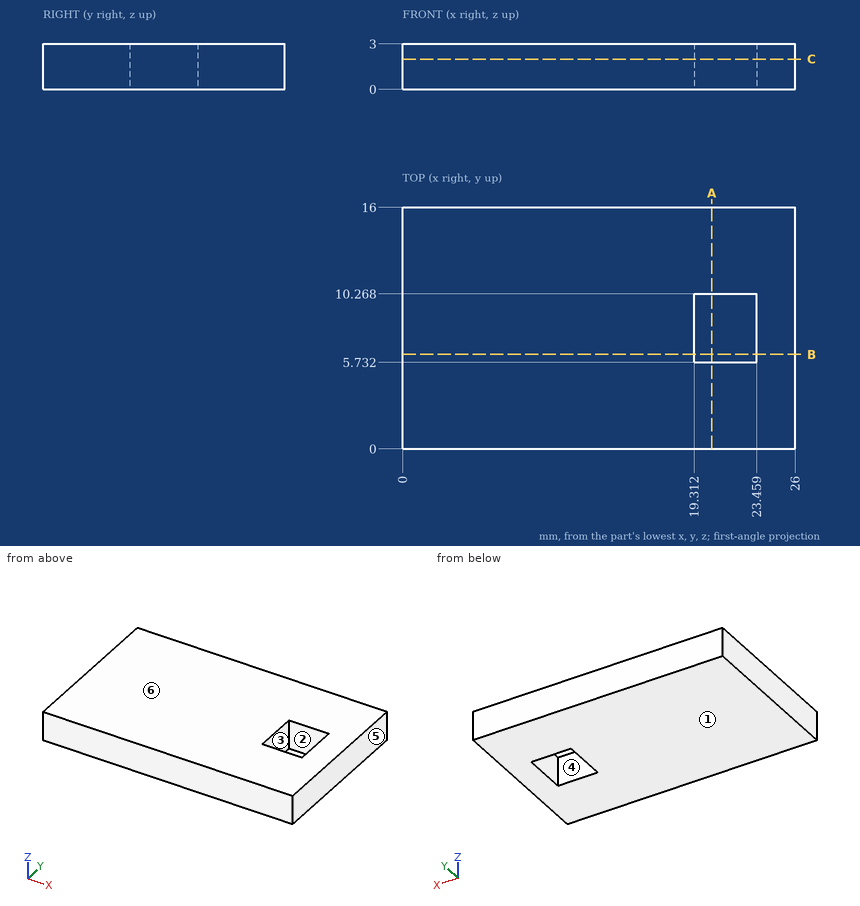
The figure shows three views and two pictorial views of one solid part (mm, origin at its lowest corner). Answer the questions. A direction names the side the tool comes from. Give positions to 0.01 mm unless a question says otherwise; leave off trailing zeros. Write each loop counter-clockwise with the first axis right and the second up, starting at its lowest first coordinate (ties: lowest second). Pieces come first, ordered by that corner, then holes. Notation, with made-up numbers: M 7,43 L 34,43 A25 cw 34,81 Z; hole C -9,71.5 d5. An arc over 180 degrees is marked long. One line per item, written item: value. Start each with the question number.
(1) A tool of negligible diameter and unlimited length cuts with its end or side. For the marked faces 1 and 2, from which of +Z, -Z, +X, -X, +Y, -Y can it reach the whole face along a straight path? Write none if from no direction.
(2) Find section C-C (z = 2). Determine the outline of the cut face in (x, y), plus the area to 3 significant figures.
(3) Determine the mould class of the marked faces 3, 4, 5 and 6 for opening direction X: pulls with the +X half, pulls with the -X half, needs draft (parallel to the pull), parting line crosses it, or undercut.
(4) Find the intervals of material crossed by line 1 (X direction, y = 8.25, z = 0.35), in increasing order.
(5) Find section B-B (y = 6.25). Determine the outline of the cut face in (x, z).
(6) Find section A-A (x = 20.5). Determine the outline of the cut face in (y, z).
Results below:
1. face 1: -Z, +X, -X, +Y, -Y
1. face 2: +Z, -Z
2. outline: M 0,0 L 26,0 L 26,16 L 0,16 Z; hole M 19.31,5.73 L 23.46,5.73 L 23.46,10.27 L 19.31,10.27 Z
2. area: 397 mm^2
3. face 3: undercut
3. face 4: undercut
3. face 5: pulls with the +X half
3. face 6: needs draft
4. line 1: x = 0 to 19.31, 23.46 to 26
5. outline: M 0,0 L 19.31,0 L 19.31,3 L 0,3 Z; M 23.46,0 L 26,0 L 26,3 L 23.46,3 Z
6. outline: M 0,0 L 5.73,0 L 5.73,3 L 0,3 Z; M 10.27,0 L 16,0 L 16,3 L 10.27,3 Z
